from build123d import *

# Parameters (mm, degrees)
SKETCH1_R            = 3
BOSS_EXTRUDE1_DEPTH  = 8
CUT_EXTRUDE1_START   = -1
SKETCH2_R            = 3.4
SKETCH2_R_2          = 3
CUT_EXTRUDE1_DEPTH   = 1
LPATTERN1_COUNT      = 5
LPATTERN1_PITCH      = 8
LPATTERN1_COUNT_DIR2 = 2
LPATTERN1_PITCH_DIR2 = 7
CUT_EXTRUDE2_DEPTH   = 3
LPATTERN2_COUNT      = 4
LPATTERN2_PITCH      = 8
LPATTERN2_COUNT_DIR2 = 2
LPATTERN2_PITCH_DIR2 = 5


with BuildPart() as part:
    # Sketch1 → Boss-Extrude1 (new body)
    with BuildSketch(Plane(origin=(0, 0, 0), x_dir=(1, 0, 0), z_dir=(0, 1, 0))):
        with BuildLine():
            Line((0, 4), (32, 4))
            ThreePointArc((32, 4), (36, 0), (32, -4))
            Line((32, -4), (0, -4))
            ThreePointArc((0, -4), (-4, 0), (0, 4))
        make_face()
        with Locations(Location((8, 0, 0), (0, 0, 270))):
            Circle(SKETCH1_R, mode=Mode.SUBTRACT)
        with Locations(Location((16, 0, 0), (0, 0, 270))):
            Circle(SKETCH1_R, mode=Mode.SUBTRACT)
        with Locations(Location((0, 0, 0), (0, 0, 270))):
            Circle(SKETCH1_R, mode=Mode.SUBTRACT)
        with Locations(Location((24, 0, 0), (0, 0, 270))):
            Circle(SKETCH1_R, mode=Mode.SUBTRACT)
        with Locations(Location((32, 0, 0), (0, 0, 270))):
            Circle(SKETCH1_R, mode=Mode.SUBTRACT)
    extrude(amount=BOSS_EXTRUDE1_DEPTH)

    # Sketch2 → Cut-Extrude1 (cut)
    with BuildSketch(Plane(origin=(0, 8, 0), x_dir=(1, 0, 0), z_dir=(0, 1, 0)).offset(CUT_EXTRUDE1_START)):
        with Locations(Location((0, 0, 0), (0, 0, 270))):
            Circle(SKETCH2_R)
        with Locations(Location((0, 0, 0), (0, 0, 270))):
            Circle(SKETCH2_R_2, mode=Mode.SUBTRACT)
    cut_extrude1 = extrude(amount=CUT_EXTRUDE1_DEPTH, mode=Mode.SUBTRACT)

    # LPattern1: Cut-Extrude1 5 × 2
    with Locations(*[(i * LPATTERN1_PITCH, -j * LPATTERN1_PITCH_DIR2, 0) for i in range(LPATTERN1_COUNT) for j in range(LPATTERN1_COUNT_DIR2) if (i, j) != (0, 0)]):
        add(cut_extrude1, mode=Mode.SUBTRACT)

    # Sketch3 → Cut-Extrude2 (cut)
    with BuildSketch(Plane(origin=(0, 8, 0), x_dir=(1, 0, 0), z_dir=(0, 1, 0))):
        with BuildLine():
            Line((3.066679245, -3.4), (4.933320755, -3.4))
            Line((4.933320755, -3.4), (5.333320755, -2.707179677))
            ThreePointArc((5.333320755, -2.707179677), (4.2, 0), (5.333320755, 2.707179677))
            Line((5.333320755, 2.707179677), (4.933320755, 3.4))
            Line((4.933320755, 3.4), (3.066679245, 3.4))
            Line((3.066679245, 3.4), (2.666679245, 2.707179677))
            ThreePointArc((2.666679245, 2.707179677), (3.8, 0), (2.666679245, -2.707179677))
            Line((2.666679245, -2.707179677), (3.066679245, -3.4))
        make_face()
    cut_extrude2 = extrude(amount=-CUT_EXTRUDE2_DEPTH, mode=Mode.SUBTRACT)

    # LPattern2: Cut-Extrude2 4 × 2
    with Locations(*[(i * LPATTERN2_PITCH, -j * LPATTERN2_PITCH_DIR2, 0) for i in range(LPATTERN2_COUNT) for j in range(LPATTERN2_COUNT_DIR2) if (i, j) != (0, 0)]):
        add(cut_extrude2, mode=Mode.SUBTRACT)


solid = part.part
CAD build for the part. Positions are in the model's coordinates, mm. A direction names the side the tool comes from. Give positions to 0.01 mm unless a question says otherwise; leave off trailing zeros. Order: outer loops, then holes, each group sorted by start corner. A loop starts at its lowest first (then second) coordinate and runs counter-clockwise, first axis right, second up. Notation, with made-up numbers: (-6.75, 31.5) -> (3.25, 31.5) arc R19 ccw to (3.25, 67.5) -> close; hole circle Ø4 at (-29, 74.5). An arc over 180 degrees is marked (long way). Return JSON: item names as keys, results as strings.
Q1. Drill centre lines: line 1 (Z direction, x = 28.5, y = 1.25); line 2 (X direction, y = 1.25, z = 3.25); line 3 (Y direction, x = 12, z = 2.75). Where is each one in solid material? Low to high.
Working result:
{"line 1": "-4 to -3.4, -1.48 to 1.48, 3.4 to 4", "line 2": "-2.33 to 2.98, 5.02 to 10.98, 13.02 to 18.98, 21.02 to 26.98, 29.02 to 34.33", "line 3": "3 to 5"}
Q2. Mould opens along X. For faces 4 (the face through (36, 4, 0)), 5 (the face through (-4, 4, 0)), 6 (the face through (-3, 1, 1)) say: pulls with the +X half, pulls with the -X half, needs draft (parallel to the pull), parting line crosses it, or undercut.
Working result:
{"face 4": "pulls with the +X half", "face 5": "pulls with the -X half", "face 6": "undercut"}
Q3. Saw through at B-B (y = 2.5). Count the separate pieces of the cut face and the enclosed holes in it, then the cut area to 3 significant figures.
Working result:
{"separate pieces": "1", "enclosed holes": "9", "area": "128 mm²"}
Q4. Which spindle directions (+Z, -Z, +X, -X, +Y, -Y) get a long thin tool onto all of the face, cutting with end or side? Do faces 1 (the face through (13, 1, 1)), 2 (the face through (28.68, 7.49, -0.74)), 3 (the face through (8.9, 3.96, 2.86)). Say none if no direction does.
Working result:
{"face 1": "-Y", "face 2": "+Y", "face 3": "+Y, -Y"}
Q5. Saw through at A-A (x = 8). Write the cut outline in (y, z).
Working result:
{"outline": "(0, -4) -> (8, -4) -> (8, -3.4) -> (7, -3.4) -> (7, -3) -> (1, -3) -> (1, -3.4) -> (0, -3.4) -> close; (0, 3.4) -> (1, 3.4) -> (1, 3) -> (7, 3) -> (7, 3.4) -> (8, 3.4) -> (8, 4) -> (0, 4) -> close"}
Q6. Saw through at D-D (x = 14.5). Write the cut outline in (y, z).
Working result:
{"outline": "(0, -4) -> (8, -4) -> (8, -3.05) -> (7, -3.05) -> (7, -2.6) -> (1, -2.6) -> (1, -3.05) -> (0, -3.05) -> close; (0, 3.05) -> (1, 3.05) -> (1, 2.6) -> (7, 2.6) -> (7, 3.05) -> (8, 3.05) -> (8, 4) -> (0, 4) -> close"}
